from build123d import *

# Parameters (mm, degrees)
SKETCH_W        = 40.2
SKETCH_H        = 15
PAD_DEPTH       = 53
POCKET_DEPTH    = 53
SKETCH022_W     = 26.5
SKETCH022_H     = 2
PAD015_DEPTH    = 53
SKETCH023_W     = 5.8
SKETCH023_H     = 5.8
SKETCH023_W_2   = 7
SKETCH023_H_2   = 7
POCKET007_DEPTH = 2.001
SKETCH024_W     = 6.2
SKETCH024_H     = 6.2
SKETCH024_W_2   = 8
SKETCH024_H_2   = 8
POCKET008_DEPTH = 1
SKETCH025_W     = 17.5
SKETCH025_H     = 12
POCKET009_DEPTH = 2.001
SKETCH026_R     = 1.7
POCKET010_DEPTH = 8


with BuildPart() as part:
    # Sketch → Pad (new body)
    with BuildSketch(Plane.XZ):
        with Locations((18.1, 1)):
            Rectangle(SKETCH_W, SKETCH_H)
    extrude(amount=-PAD_DEPTH)

    # Sketch001 → Pocket (cut)
    with BuildSketch(Plane.XZ):
        Polygon((-2, 11), (-2, 3), (2, 3), (2, 1), (-0.4, 1), (-0.4, 0), (0.5, 0), (0.5, -1.5), (4, -1.5), (4, -3.45), (8.5, -3.45), (8.5, -2.9), (28.85, -2.9), (28.85, -4), (35.85, -4), (35.85, 0), (36.6, 0), (36.6, 1), (35.8, 1), (35.8, 4.7), (34.6, 4.7), (34.6, 5.7), (32.6, 5.7), (32.6, 11), align=None)
    extrude(amount=-POCKET_DEPTH, mode=Mode.SUBTRACT)

    # Sketch022 → Pad015 (join)
    with BuildSketch(Plane.XZ):
        with Locations((24.95, 9.5)):
            Rectangle(SKETCH022_W, SKETCH022_H)
    extrude(amount=-PAD015_DEPTH)

    # Sketch023 → Pocket007 (cut, through all)
    with BuildSketch(Plane.XY.offset(8.5)):
        with Locations((15.2, 19)):
            Rectangle(SKETCH023_W, SKETCH023_H)
        with Locations((29.2, 19)):
            Rectangle(SKETCH023_W_2, SKETCH023_H_2)
        with Locations((15.2, 46)):
            Rectangle(SKETCH023_W, SKETCH023_H)
        with Locations((29.2, 46)):
            Rectangle(SKETCH023_W_2, SKETCH023_H_2)
    extrude(amount=POCKET007_DEPTH, mode=Mode.SUBTRACT)

    # Sketch024 → Pocket008 (cut)
    with BuildSketch(Plane.XY.offset(8.5)):
        with Locations((15.2, 19)):
            Rectangle(SKETCH024_W, SKETCH024_H)
        with Locations((29.2, 19)):
            Rectangle(SKETCH024_W_2, SKETCH024_H_2)
        with Locations((15.2, 46)):
            Rectangle(SKETCH024_W, SKETCH024_H)
        with Locations((29.2, 46)):
            Rectangle(SKETCH024_W_2, SKETCH024_H_2)
    extrude(amount=POCKET008_DEPTH, mode=Mode.SUBTRACT)

    # Sketch025 → Pocket009 (cut, through all)
    with BuildSketch(Plane.XY.offset(8.5)):
        with Locations((22.2, 32.5)):
            Rectangle(SKETCH025_W, SKETCH025_H)
    extrude(amount=POCKET009_DEPTH, mode=Mode.SUBTRACT)

    # Sketch026 → Pocket010 (cut, symmetric)
    with BuildSketch(Plane(origin=(0, 32.5, 8.5), x_dir=(1, 0, 0), z_dir=(0, -1, 0))):
        with Locations((22.2, 0)):
            Circle(SKETCH026_R)
    extrude(amount=POCKET010_DEPTH, both=True, mode=Mode.SUBTRACT)


solid = part.part
Source: CAD feature listing. Evaluate the final solid. Frame: model axes, mm. A direction names the side the tool comes from. Give positions to 0.01 mm unless a question says otherwise; leave off trailing zeros. Write each loop counter-clockwise with the first axis right and the second up, starting at its lowest first coordinate (ties: lowest second). Pieces come first, ordered by that corner, then holes. Notation, with made-up numbers: M 4.25,58 L 8.25,58 A36 ccw 8.25,97 Z; hole C -23.5,-15 d6. An arc over 180 degrees is marked long. Return JSON: item names as keys, results as strings. Group by question number.
1) Cut plane D-D, the plane z = 6.5. Output: boundary loops of the cut face in (x, y).
2) Cut plane A-A, the plane x = 22.2. Output: boundary loops of the cut face in (y, z).
3) Ray query, L1, parallel to Z at x = 36, y = 15.5; L2, parallel to X at y = 50, z = -0.25; L3, parallel to Z at x = 19, y = 4. Return the intervals inside material, ascending.
4) Draft query along Z for faces 1 (the face through (25, 26, 10.5)), 2 (the face through (22, 24.5, 9)), 3 (the face through (22, 53, -4)). Return one class per face: released by +Z, released by -Z, zero draft, split by the parting line, or undercut.
5) Set-up query: faces 4 (the face through (22.2, 25.5, 10.2)), 5 (the face through (20, 26.5, 9)), 6 (the face through (35, 26, 4.7)), 7 (the face through (4, 26, -2)), 8 (the face through (2, 26, -1.5)). Return all of +Z, -Z, +X, -X, +Y, -Y with unobstructed straight access to the full face (end or side cutting, diameter ignored); none if empty.
6) First-contact query: pin 1 Ø1.3 at (x, y) = (6.5, 33.5) entering from +Z; pin 2 Ø0.6 at (y, z) = (33, 10) entering from -X; pin 3 Ø2 at (x, y) = (0.5, 35) entering from +Z. Flat tips, straight axial feed; report the tip coordinate or a pass-through.
Data:
{
 "1": {"outline": "M 32.6,0 L 38.2,0 L 38.2,53 L 32.6,53 Z"},
 "2": {"outline": "M 0,-6.5 L 53,-6.5 L 53,-2.9 L 0,-2.9 Z; M 0,8.5 L 24.5,8.5 L 24.5,10.2 L 26.5,10.2 L 26.5,10.5 L 0,10.5 Z; M 38.5,10.2 L 40.5,10.2 L 40.5,8.5 L 53,8.5 L 53,10.5 L 38.5,10.5 Z"},
 "3": {"L1": "z = -6.5 to 0, 1 to 10.5", "L2": "x = -2 to 0.5, 35.85 to 38.2", "L3": "z = -6.5 to -2.9, 8.5 to 10.5"},
 "4": {"face 1": "released by +Z", "face 2": "undercut", "face 3": "zero draft"},
 "5": {"face 4": "none", "face 5": "+Z", "face 6": "-X, +Y, -Y", "face 7": "+Z, +Y, -Y", "face 8": "+Y, -Y"},
 "6": {"pin 1": "stops at z = -3.45", "pin 2": "stops at x = 11.7", "pin 3": "stops at z = 3"}
}
